from build123d import *

# Parameters (mm, degrees)
SKETCH1_R           = 2.38125
BOSS_EXTRUDE1_DEPTH = 5.842
FILLET1_R           = 3.175
FILLET2_R           = 3.175
FILLET3_R           = 1.5875
FILLET5_R           = 6.35


with BuildPart() as part:
    # Sketch1 → Boss-Extrude1 (new body)
    with BuildSketch(Plane(origin=(0, 0, 0), x_dir=(1, 0, 0), z_dir=(0, 1, 0))):
        Polygon((-11.01238397, -123.675577549), (12.699883629, -68.919434524), (33.84630657, 4.876477372), (21.14630657, 26.873522628), (-33.84630657, -4.876477372), (-27.49630657, -15.875), (-61.093499563, -49.937045256), (-22.993499563, -115.928181024), (-33.992022192, -122.278181024), (-30.325847982, -128.628181024), (-22.010906598, -130.025577549), align=None)
        with Locations(Location((21.997045256, 12.7, 0), (0, 0, 270))):
            Circle(SKETCH1_R, mode=Mode.SUBTRACT)
        with Locations(Location((10.998522628, 6.35, 0), (0, 0, 270))):
            Circle(SKETCH1_R, mode=Mode.SUBTRACT)
        with Locations(Location((0, 0, 0), (0, 0, 270))):
            Circle(SKETCH1_R, mode=Mode.SUBTRACT)
        with Locations(Location((-10.998522628, -6.35, 0), (0, 0, 270))):
            Circle(SKETCH1_R, mode=Mode.SUBTRACT)
        with Locations(Location((-21.997045256, -12.7, 0), (0, 0, 270))):
            Circle(SKETCH1_R, mode=Mode.SUBTRACT)
        with Locations(Location((0, -24.4695218, 0), (0, 0, 270))):
            Circle(SKETCH1_R, mode=Mode.SUBTRACT)
        with Locations(Location((0, -37.1695218, 0), (0, 0, 270))):
            Circle(SKETCH1_R, mode=Mode.SUBTRACT)
        with Locations(Location((0, -49.8695218, 0), (0, 0, 270))):
            Circle(SKETCH1_R, mode=Mode.SUBTRACT)
        with Locations(Location((0, -62.5695218, 0), (0, 0, 270))):
            Circle(SKETCH1_R, mode=Mode.SUBTRACT)
        with Locations(Location((0, -75.2695218, 0), (0, 0, 270))):
            Circle(SKETCH1_R, mode=Mode.SUBTRACT)
        Polygon((25.931282224, 0.306735935), (12.7, -7.332348419), (12.7, -16.277642723), (12.7, -45.867554067), align=None, mode=Mode.SUBTRACT)
        Polygon((-43.744976935, -54.585567884), (-37.571232702, -65.27880657), (-19.05, -54.585567884), align=None, mode=Mode.SUBTRACT)
        Polygon((-12.7, -22.427495922), (-12.7, -46.106477151), (-18.344976935, -46.106477151), (-38.267154833, -46.106477151), (-18.344976935, -27.655582651), align=None, mode=Mode.SUBTRACT)
        Polygon((-18.344976935, -98.579658396), (-12.7, -108.357045256), (-12.7, -101.6), (-12.7, -58.251742094), (-34.396232702, -70.778067884), align=None, mode=Mode.SUBTRACT)
    extrude(amount=BOSS_EXTRUDE1_DEPTH)

    # Fillet1
    fillet1_edges = [part.edges().sort_by_distance(p)[0] for p in [
        (-19.05, 2.921, 54.585567884),
        (-43.744976935, 2.921, 54.585567884),
        (-37.571232702, 2.921, 65.27880657),
        (12.7, 2.921, 7.332348419),
        (12.7, 2.921, 45.867554067),
        (25.931282224, 2.921, -0.306735935),
        (-34.396232702, 2.921, 70.778067884),
        (-12.7, 2.921, 108.357045256),
        (-12.7, 2.921, 58.251742094),
        (-12.7, 2.921, 46.106477151),
        (-12.7, 2.921, 22.427495922),
        (-38.267154833, 2.921, 46.106477151),
    ]]
    fillet(fillet1_edges, radius=FILLET1_R)

    # Fillet2
    fillet2_edges = [part.edges().sort_by_distance(p)[0] for p in [
        (-33.84630657, 2.921, 4.876477372),
        (21.14630657, 2.921, -26.873522628),
        (33.84630657, 2.921, -4.876477372),
        (-61.093499563, 2.921, 49.937045256),
        (-27.49630657, 2.921, 15.875),
    ]]
    fillet(fillet2_edges, radius=FILLET2_R)

    # Fillet3
    fillet3_edges = [part.edges().sort_by_distance(p)[0] for p in [
        (-33.992022192, 2.921, 122.278181024),
        (-22.993499563, 2.921, 115.928181024),
    ]]
    fillet(fillet3_edges, radius=FILLET3_R)

    # Fillet5
    fillet5_edges = [part.edges().sort_by_distance(p)[0] for p in [
        (12.699883629, 2.921, 68.919434524),
        (-11.01238397, 2.921, 123.675577549),
        (-22.010906598, 2.921, 130.025577549),
        (-30.325847982, 2.921, 128.628181024),
    ]]
    fillet(fillet5_edges, radius=FILLET5_R)


solid = part.part
Verification items for the finished model (mm, model axes). A direction names the side the tool comes from. Give positions to 0.01 mm unless a question says otherwise; leave off trailing zeros. Write each loop counter-clockwise with the first axis right and the second up, starting at its lowest first coordinate (ties: lowest second). Pieces come first, ordered by that corner, then holes.
(1) Access from +Z, -Z, +X, -X, +Y, -Y to the whole of each face (thin tool, end or side, straight path). Record for faces 1 (the face through (16.74, 2.88, 5)), 2 (the face through (-42.088, 2.88, 82.855)), 3 (the face through (-14, 0, 51)).
(2) Cross-section at D-D (x = -51). Enter the section's corners in (y, z), plus the area to 3 significant figures.
(3) Cross-section at B-B (x = 0). Enter the section's corners in (y, z), plus the area to 3 significant figures.
(4) Mould release check, pull along Z, two halves, no side actions. Record for faces 4 (the face through (-60.28, 2.96, 50.01)), 5 (the face through (-14, 5.842, 51)), 6 (the face through (-9.389, 2.88, 4.595)): +Z half, -Z half, draft (parallel to the pull), parting line (faces both ways), or undercut.
(5) Gauge pin test, flat ends, axial feed: pin 1 (5.5 mm diameter, centred on x = 0, z = 0, fed in from +Y); pin 2 (1.5 mm diameter, centred on x = -17, y = 1, fed in from +Z); pin 3 (3 mm diameter, centred on x = -35, y = 3, fed in from +Z); pin 4 (1 mm diameter, centred on y = 4, z = 8.5, fed in from -X). Record the tip position at first contact, or that the pin passes through.
(6) Material ranges on line 1 (X direction, y = 3.2, z = 12.7); line 2 (X direction, y = 2.8, z = 24); line 3 (Z direction, x = -30.5, y = 3), recorded low to high.
(7) Cross-section at A-A (z = 0). Enter the section's corners in (x, y).
(8) Cross-section at C-C (y = 2.9). State how many separate pieces and enclosed holes the cut face has, plus the area to 3 significant figures.
Worked out:
1. face 1: +Y, -Y
1. face 2: -X, +Y, -Y
1. face 3: +Z, -Z, +X, -X, -Y
2. outline: (0, 39.7) - (5.84, 39.7) - (5.84, 67.42) - (0, 67.42) - close
2. area: 162 mm2
3. outline: (0, -14.66) - (5.84, -14.66) - (5.84, -2.38) - (0, -2.38) - close; (0, 2.38) - (5.84, 2.38) - (5.84, 22.09) - (0, 22.09) - close; (0, 26.85) - (5.84, 26.85) - (5.84, 34.79) - (0, 34.79) - close; (0, 39.55) - (5.84, 39.55) - (5.84, 47.49) - (0, 47.49) - close; (0, 52.25) - (5.84, 52.25) - (5.84, 60.19) - (0, 60.19) - close; (0, 64.95) - (5.84, 64.95) - (5.84, 72.89) - (0, 72.89) - close; (0, 77.65) - (5.84, 77.65) - (5.84, 98.25) - (0, 98.25) - close
3. area: 493 mm2
4. face 4: parting line
4. face 5: draft
4. face 6: undercut
5. pin 1: stops at y = 5.84
5. pin 2: stops at z = 127.57
5. pin 3: stops at z = 97.73
5. pin 4: stops at x = -32.04
6. line 1: x = -29.33 to -24.38, -19.62 to 12.7, 22.2 to 28.81
6. line 2: x = -35.51 to -2.33, 2.33 to 12.79, 18.97 to 25.57
6. line 3: z = 2.94 to 10.67, 18.92 to 38.91, 46.09 to 54.61, 61.2 to 68.53, 77.53 to 102.93, 120.26 to 127.64
7. outline: (-25.4, 0) - (-2.38, 0) - (-2.38, 5.84) - (-25.4, 5.84) - close; (2.38, 0) - (32.45, 0) - (32.45, 5.84) - (2.38, 5.84) - close
8. separate pieces: 1
8. enclosed holes: 14
8. area: 6,250 mm2
